```python
from build123d import *

# Parameters (mm, degrees)
F0_W     = 137
F0_H     = 91.5
F1_DEPTH = 30
F2_W     = 127
F2_H     = 81.5
F3_DEPTH = 25
F4_W     = 25
F4_H     = 20
F4_W_2   = 14
F4_W_3   = 26.5
F5_DEPTH = 5


with BuildPart() as f1:
    # F0 (on Top) → F1 (new body)
    with BuildSketch(Plane.XY):
        with Locations((-5.744236, 11.116833)):
            Rectangle(F0_W, F0_H)
    extrude(amount=F1_DEPTH)

    # F2 (on face) → F3 (cut)
    with BuildSketch(Plane.XY.offset(30)):
        with Locations((-5.744236, 11.116833)):
            Rectangle(F2_W, F2_H)
    extrude(amount=-F3_DEPTH, mode=Mode.SUBTRACT)

    # F4 (on face) → F5 (cut)
    with BuildSketch(Plane.YZ.offset(62.755764)):
        with Locations((-17.133167, 15)):
            Rectangle(F4_W, F4_H)
        with Locations((6.366833, 15)):
            Rectangle(F4_W_2, F4_H)
        with Locations((38.616833, 15)):
            Rectangle(F4_W_3, F4_H)
    extrude(amount=-F5_DEPTH, mode=Mode.SUBTRACT)


solid = f1.part
```
For this review, take the finished solid that the model builds, in its own axes (mm). A direction names the side the tool comes from. Coordinates: 2 decimals unless noted, no trailing zeros. Write each loop counter-clockwise with the first axis right and the second up, starting at its lowest first coordinate (ties: lowest second). Pieces come first, ordered by that corner, then holes. Notation, with made-up numbers: (-36, 12.25) - (-14, 12.25) arc R26 ccw to (-14, 39.25) - close; hole circle Ø9 at (80.5, -26.75). An arc over 180 degrees is marked (long way). Answer in a Markdown table with one row per item. Add a question column.
Q1. For probe 1 along Y at (x, z) = (-1.5, 7.75); probe 2 along X at (y, z) = (-11.5, 28); probe 3 along Z at (x, y) = (53, 16), list the stretches that pass through material, from the lowest coordinate up.
Q2. We need section B-B, the plane y = 38.5. State the section outline as (x, z) points.
Q3. Draft analysis for pull direction X (two halves, no side actions). For faces 4 (the flat face through (57.756, 14, 21)), 5 (the flat face through (60, -17, 25)), 6 (the flat face through (62.756, 10.5, 4.8)), state which applies: +X half, -X half, draft (parallel to the pull), parting line (faces both ways), or undercut.
Q4. We need section C-C, the plane x = 33.5. State the section outline as (y, z) points.
Q5. For P1, Ø1, axis at x = 36.5, y = 36, coming from the -Z side, flat-tipped, find the tip position at first contact; note if it passes through.
Q6. We need section A-A, the plane z = 7. State the section outline as (x, y) points.
Q7. We need section D-D, the plane z = 27.5. State the section outline as (x, y) points.
Q8. Tool access review of faces 1 (the flat face through (60, 13.367, 15)), 2 (the flat face through (-69.244, 11, 18)), 3 (the flat face through (-7, 12, 0)): name each direction out of +Z, -Z, +X, -X, +Y, -Y from which nothing blocks a thin tool from reaching the whole face with its end or side.
Answer list:
| question | item | result |
|---|---|---|
| 1 | probe 1 | y = -34.63 to -29.63, 51.87 to 56.87 |
| 1 | probe 2 | x = -74.24 to -69.24, 57.76 to 62.76 |
| 1 | probe 3 | z = 0 to 5 |
| 2 | outline | (-74.24, 0) - (62.76, 0) - (62.76, 5) - (-69.24, 5) - (-69.24, 30) - (-74.24, 30) - close; (57.76, 25) - (62.76, 25) - (62.76, 30) - (57.76, 30) - close |
| 3 | face 4 | undercut |
| 3 | face 5 | draft |
| 3 | face 6 | +X half |
| 4 | outline | (-34.63, 0) - (56.87, 0) - (56.87, 30) - (51.87, 30) - (51.87, 5) - (-29.63, 5) - (-29.63, 30) - (-34.63, 30) - close |
| 5 | P1 | stops at z = 0 |
| 6 | outline | (-74.24, -34.63) - (62.76, -34.63) - (62.76, -29.63) - (-69.24, -29.63) - (-69.24, 51.87) - (62.76, 51.87) - (62.76, 56.87) - (-74.24, 56.87) - close; (57.76, -4.63) - (62.76, -4.63) - (62.76, -0.63) - (57.76, -0.63) - close; (57.76, 13.37) - (62.76, 13.37) - (62.76, 25.37) - (57.76, 25.37) - close |
| 7 | outline | (-74.24, -34.63) - (62.76, -34.63) - (62.76, 56.87) - (-74.24, 56.87) - close; hole (-69.24, -29.63) - (57.76, -29.63) - (57.76, 51.87) - (-69.24, 51.87) - close |
| 8 | face 1 | +X |
| 8 | face 2 | +Z |
| 8 | face 3 | -Z, +X, -X, +Y, -Y |
